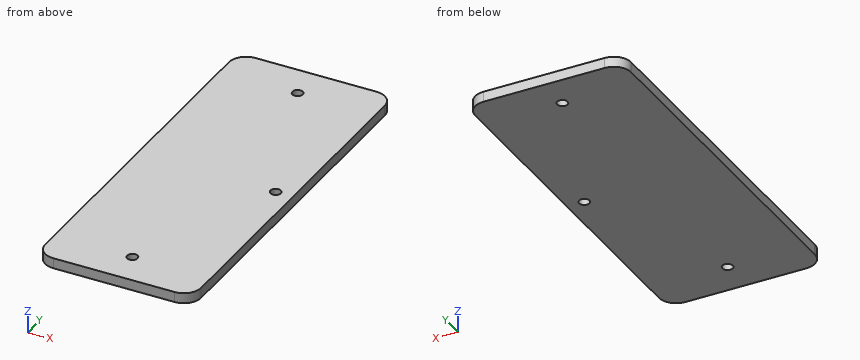
```python
from build123d import *

# Parameters (mm, degrees)
SKETCH1_R           = 1.5
BOSS_EXTRUDE1_DEPTH = 3
SKETCH4_R           = 1.5
CUT_EXTRUDE1_DEPTH  = 60.5


with BuildPart() as part:
    # Sketch1 → Boss-Extrude1 (new body)
    with BuildSketch(Plane.XY):
        with BuildLine():
            Line((-17.5, 55), (17.5, 55))
            ThreePointArc((17.5, 55), (21.035533906, 53.535533906), (22.5, 50))
            Line((22.5, 50), (22.5, -50))
            ThreePointArc((22.5, -50), (21.035533906, -53.535533906), (17.5, -55))
            Line((17.5, -55), (-17.5, -55))
            ThreePointArc((-17.5, -55), (-21.035533906, -53.535533906), (-22.5, -50))
            Line((-22.5, -50), (-22.5, 50))
            ThreePointArc((-22.5, 50), (-21.035533906, 53.535533906), (-17.5, 55))
        make_face()
        with Locations((17.5, 0)):
            Circle(SKETCH1_R, mode=Mode.SUBTRACT)
    extrude(amount=BOSS_EXTRUDE1_DEPTH)

    # Sketch4 → Cut-Extrude1 (cut, through all)
    with BuildSketch(Plane.XY.offset(3)):
        with Locations((0, 45)):
            Circle(SKETCH4_R)
        with Locations((0, -45)):
            Circle(SKETCH4_R)
    extrude(amount=-CUT_EXTRUDE1_DEPTH, mode=Mode.SUBTRACT)


solid = part.part
```
The model under review builds one solid part; all positions refer to its coordinate system, in mm. Coordinates: 2 decimals unless noted, no trailing zeros. Order: outer loops, then holes, each group sorted by start corner. A loop starts at its lowest first (then second) coordinate and runs counter-clockwise, first axis right, second up. Notation, with made-up numbers: (80.25, 2.5) -> (109.25, 2.5) arc R26 ccw to (109.25, 36.5) -> close; hole circle Ø10 at (-22, -20). An arc over 180 degrees is marked (long way). Answer in a Markdown table with one row per item. Add a question column.
Item 1: We need section A-A on y = 45. Write out the cut boundary in (x, z).
Item 2: Clearance check with flat-ended pins moving along their axes: pin 1 (5 mm diameter, centred on x = 0, y = -45, fed in from -Z); pin 2 (2.5 mm diameter, centred on x = 17.5, y = 0, fed in from +Z). State where each tip first meets the part, or that it passes through.
Item 3: We need section B-B on x = 0. Write out the cut boundary in (y, z).
Item 4: To check wall thickness, follow probe 1 along Y at (x, z) = (0, 1.15); probe 2 along Y at (x, z) = (-21, 2.55); probe 3 along Y at (x, z) = (21.5, 0.45). State the ranges of each line that lie inside material, in increasing order.
Final values:
| question | item | result |
|---|---|---|
| 1 | outline | (-22.5, 0) -> (-1.5, 0) -> (-1.5, 3) -> (-22.5, 3) -> close; (1.5, 0) -> (22.5, 0) -> (22.5, 3) -> (1.5, 3) -> close |
| 2 | pin 1 | stops at z = 0 |
| 2 | pin 2 | passes through |
| 3 | outline | (-55, 0) -> (-46.5, 0) -> (-46.5, 3) -> (-55, 3) -> close; (-43.5, 0) -> (43.5, 0) -> (43.5, 3) -> (-43.5, 3) -> close; (46.5, 0) -> (55, 0) -> (55, 3) -> (46.5, 3) -> close |
| 4 | probe 1 | y = -55 to -46.5, -43.5 to 43.5, 46.5 to 55 |
| 4 | probe 2 | y = -53.57 to 53.57 |
| 4 | probe 3 | y = -53 to 53 |
